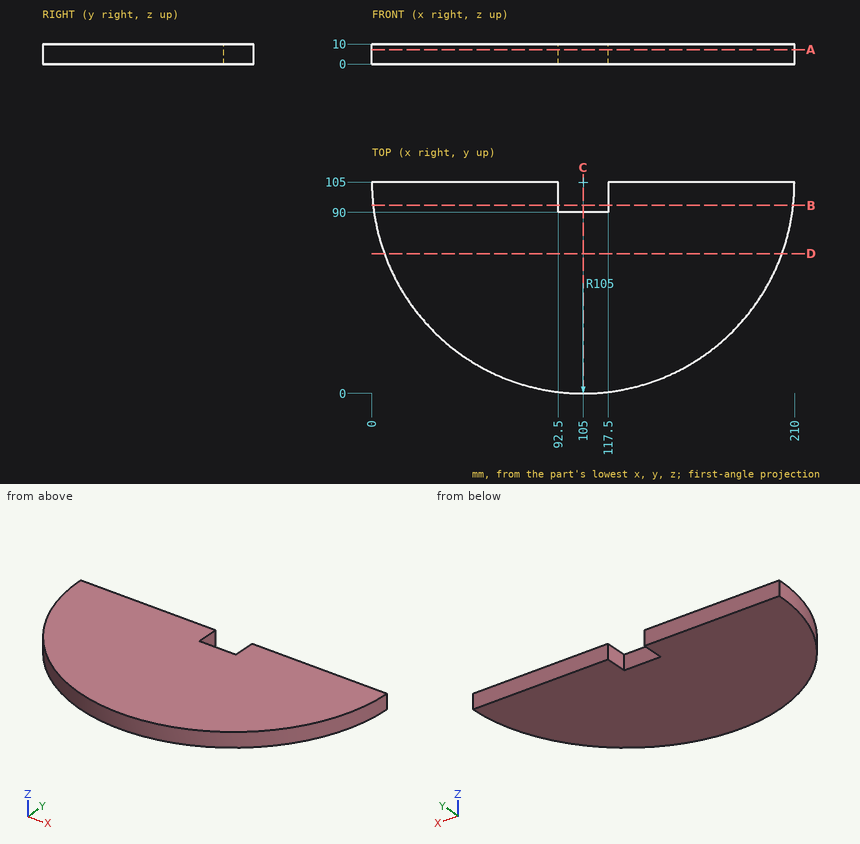
Job drawing, mm, ordinate dimensions from the low corner. One solid piece. Round coordinates to 2 decimals unless told otherwise and drop trailing zeros. Write each loop counter-clockwise with the first axis right and the second up, starting at its lowest first coordinate (ties: lowest second). Pieces come first, ordered by that corner, then holes. Notation, with made-up numbers: M -27,-35 L 14,-35 A23 ccw 14,-14 Z; hole C -27.5,80 d8. An arc over 180 degrees is marked long. Return JSON: item names as keys, results as strings. Group by question number.
(1) Pin check, flat tips, straight feed: pin 1 Ø2 at (x, z) = (79, 1) entering from -Y; pin 2 Ø5 at (y, z) = (94, 3.5) entering from -X; pin 3 Ø1 at (y, z) = (19.5, 1.5) entering from -X. Stop position of each tip, or through.
(2) Drill centre lines: probe 1 along X at (y, z) = (93, 4.75); probe 2 along Y at (x, z) = (178.5, 9.75) (3 decimals); probe 3 along X at (y, z) = (78.5, 9.25). Where is each one in solid material? Low to high.
(3) Saw through at B-B on y = 93.5. Write the cut outline in (x, z), then the cut area to 3 significant figures.
(4) Saw through at A-A on z = 7.25. Write the cut outline in (x, y), then the cut area to 3 significant figures.
(5) Saw through at D-D on y = 69.5. Write the cut outline in (x, z), then the cut area to 3 significant figures.
(6) Saw through at C-C on x = 105. Write the cut outline in (y, z).
Returned:
{
 "1": {"pin 1": "y = 3.02", "pin 2": "x = 0.34", "pin 3": "x = 43.36"},
 "2": {"probe 1": "0.69 to 92.5, 117.5 to 209.31", "probe 2": "30.015 to 105", "probe 3": "3.4 to 206.6"},
 "3": {"outline": "M 0.63,0 L 92.5,0 L 92.5,10 L 0.63,10 Z; M 117.5,0 L 209.37,0 L 209.37,10 L 117.5,10 Z", "area": "1,840 mm²"},
 "4": {"outline": "M 0,105 A105 ccw 210,105 L 117.5,105 L 117.5,90 L 92.5,90 L 92.5,105 Z", "area": "16,900 mm²"},
 "5": {"outline": "M 6.18,0 L 203.82,0 L 203.82,10 L 6.18,10 Z", "area": "1,980 mm²"},
 "6": {"outline": "M 0,0 L 90,0 L 90,10 L 0,10 Z"}
}
